Verification items for the finished model (mm, model axes). A direction names the side the tool comes from. Round coordinates to 2 decimals unless told otherwise and drop trailing zeros. Write each loop counter-clockwise with the first axis right and the second up, starting at its lowest first coordinate (ties: lowest second). Pieces come first, ordered by that corner, then holes. Notation, with made-up numbers: (-36.5, -10.5) - (8.5, -10.5) arc R27 ccw to (8.5, 24.5) - close; hole circle Ø4 at (-13, 25.5). An arc over 180 degrees is marked (long way). Answer as a JSON object with one key per item and string values.
```python
from build123d import *

# Parameters (mm, degrees)
F1_DEPTH = 13
F2_DEPTH = 6


with BuildPart() as f1:
    # F0 (on Top) → F1 (new body)
    with BuildSketch(Plane.XY):
        with BuildLine():
            Line((-128.226717, 65.178408), (-128.095499, -75.93241))
            Line((-128.095499, -75.93241), (113.904396, -75.707376))
            Line((113.904396, -75.707376), (113.770597, 68.1803))
            ThreePointArc((113.770597, 68.1803), (111.089038, 74.581091), (104.650671, 77.171132))
            Line((104.650671, 77.171132), (-119.34665, 74.185978))
            ThreePointArc((-119.34665, 74.185978), (-125.635881, 71.505215), (-128.226717, 65.178408))
        make_face()
        with BuildLine():
            Line((92.904501, -63.93241), (-104.095499, -63.93241))
            ThreePointArc((-104.095499, -63.93241), (-110.45946, -61.296371), (-113.095499, -54.93241))
            Line((-113.095499, -54.93241), (-113.095499, 52.06759))
            ThreePointArc((-113.095499, 52.06759), (-110.45946, 58.431551), (-104.095499, 61.06759))
            Line((-104.095499, 61.06759), (92.904501, 61.06759))
            ThreePointArc((92.904501, 61.06759), (99.268462, 58.431551), (101.904501, 52.06759))
            Line((101.904501, 52.06759), (101.904501, -54.93241))
            ThreePointArc((101.904501, -54.93241), (99.268462, -61.296371), (92.904501, -63.93241))
        make_face(mode=Mode.SUBTRACT)
    extrude(amount=F1_DEPTH)

    # F0 (on Top) → F2 (join)
    with BuildSketch(Plane.XY):
        with BuildLine():
            ThreePointArc((-113.095499, -54.93241), (-110.45946, -61.296371), (-104.095499, -63.93241))
            Line((-104.095499, -63.93241), (92.904501, -63.93241))
            ThreePointArc((92.904501, -63.93241), (99.268462, -61.296371), (101.904501, -54.93241))
            Line((101.904501, -54.93241), (101.904501, 52.06759))
            ThreePointArc((101.904501, 52.06759), (99.268462, 58.431551), (92.904501, 61.06759))
            Line((92.904501, 61.06759), (-104.095499, 61.06759))
            ThreePointArc((-104.095499, 61.06759), (-110.45946, 58.431551), (-113.095499, 52.06759))
            Line((-113.095499, 52.06759), (-113.095499, -54.93241))
        make_face()
        with BuildLine():
            ThreePointArc((96.904501, -54.93241), (95.732928, -57.760837), (92.904501, -58.93241))
            Line((92.904501, -58.93241), (-104.095499, -58.93241))
            ThreePointArc((-104.095499, -58.93241), (-106.923927, -57.760837), (-108.0955, -54.93241))
            Line((-108.0955, -54.93241), (-108.0955, 52.06759))
            ThreePointArc((-108.0955, 52.06759), (-106.923927, 54.896018), (-104.095499, 56.067591))
            Line((-104.095499, 56.067591), (92.904501, 56.067591))
            ThreePointArc((92.904501, 56.067591), (95.732928, 54.896018), (96.904501, 52.06759))
            Line((96.904501, 52.06759), (96.904501, -54.93241))
        make_face(mode=Mode.SUBTRACT)
    extrude(amount=F2_DEPTH)


solid = f1.part
```
1. Cross-section at B-B (z = 10). Record the boundary of the cut face in (x, y), plus the area to 3 significant figures.
Completed:
{"outline": "(-128.23, 65.18) - (-128.1, -75.93) - (113.9, -75.71) - (113.77, 68.18) arc R9 ccw to (104.65, 77.17) - (-119.35, 74.19) arc R9 ccw to start; hole (-113.1, -54.93) arc R9 ccw to (-104.1, -63.93) - (92.9, -63.93) arc R9 ccw to (101.9, -54.93) - (101.9, 52.07) arc R9 ccw to (92.9, 61.07) - (-104.1, 61.07) arc R9 ccw to (-113.1, 52.07) - close", "area": "9,820 mm^2"}
2. Go/stop test with flat-tipped pins: pin 1 (2 mm diameter, centred on y = -20.5, z = 7.5, fed in from -X); pin 2 (5.5 mm diameter, centred on x = -30, z = 9.5, fed in from -Y); pin 3 (1 mm diameter, centred on y = 3, z = 5.5, fed in from -X). Record where each tip stops, or that it passes through.
Completed:
{"pin 1": "stops at x = -128.15", "pin 2": "stops at y = -75.84", "pin 3": "stops at x = -128.17"}
3. Access from +Z, -Z, +X, -X, +Y, -Y to the whole of each face (thin tool, end or side, straight path). Record for faces 4 (the face through (99.2, 58.5, 9.5)), 5 (the face through (-17, 63, 13)), 6 (the face through (-4, -58.932, 3)).
Completed:
{"face 4": "+Z", "face 5": "+Z, +X, -X, +Y, -Y", "face 6": "+Z, -Z"}
4. Cross-section at C-C (y = 6). Record the boundary of the cut face in (x, z).
Completed:
{"outline": "(-128.17, 0) - (-108.1, 0) - (-108.1, 6) - (-113.1, 6) - (-113.1, 13) - (-128.17, 13) - close; (96.9, 0) - (113.83, 0) - (113.83, 13) - (101.9, 13) - (101.9, 6) - (96.9, 6) - close"}
5. Mould release check, pull along Y, two halves, no side actions. Record for faces 1 (the face through (-7, 61.068, 9)), 2 (the face through (-9, -66, 0)), 3 (the face through (111.16, 74.51, 6.41)): released by +Y, released by -Y, zero draft, split by the parting line, or undercut.
Completed:
{"face 1": "undercut", "face 2": "zero draft", "face 3": "released by +Y"}
6. Material ranges on probe 1 along X at (y, z) = (25, 7.5); probe 2 along X at (y, z) = (19.5, 4); probe 3 along Y at (x, z) = (102, 10.5), recorded low to high. Write a range as from..to.
Completed:
{"probe 1": "x = -128.19..-113.1, 101.9..113.81", "probe 2": "x = -128.18..-108.1, 96.9..113.82", "probe 3": "y = -75.72..77.14"}
7. Cross-section at A-A (x = 31.5). Record the boundary of the cut face in (y, z), plus the area to 3 significant figures.
Completed:
{"outline": "(-75.78, 0) - (-58.93, 0) - (-58.93, 6) - (-63.93, 6) - (-63.93, 13) - (-75.78, 13) - close; (56.07, 0) - (76.2, 0) - (76.2, 13) - (61.07, 13) - (61.07, 6) - (56.07, 6) - close", "area": "411 mm^2"}
